```python
from build123d import *

# Parameters (mm, degrees)
F0_W      = 42
F0_H      = 13
F1_DEPTH  = 6
F2_W      = 17
F2_H      = 13
F5_DEPTH  = 27
F3_R      = 2.5
F6_DEPTH  = 6
F4_R      = 2.5
F7_DEPTH  = 6
F8_R      = 4
F9_DEPTH  = 15
F10_R     = 3.5
F11_DEPTH = 20
F12_W     = 1
F12_H     = 13
F13_DEPTH = 13


with BuildPart() as f1:
    # F0 (on Top) → F1 (new body)
    with BuildSketch(Plane.XY):
        Rectangle(F0_W, F0_H)
    extrude(amount=-F1_DEPTH)

    # F2 (on Top) → F5 (join)
    with BuildSketch(Plane.XY):
        Rectangle(F2_W, F2_H)
    extrude(amount=F5_DEPTH)

    # F3 (on Top) → F6 (cut)
    with BuildSketch(Plane.XY):
        with Locations((14.75, 0)):
            Circle(F3_R)
    extrude(amount=-F6_DEPTH, mode=Mode.SUBTRACT)

    # F4 (on Top) → F7 (cut)
    with BuildSketch(Plane.XY):
        with Locations((-14.75, 0)):
            Circle(F4_R)
    extrude(amount=-F7_DEPTH, mode=Mode.SUBTRACT)

    # F8 (on face) → F9 (cut)
    with BuildSketch(Plane.XZ.offset(6.5)):
        with Locations((0, 13.5)):
            Circle(F8_R)
    extrude(amount=-F9_DEPTH, mode=Mode.SUBTRACT)

    # F10 (on face) → F11 (cut)
    with BuildSketch(Plane.YZ.offset(8.5)):
        with Locations((0, 19)):
            Circle(F10_R)
    extrude(amount=-F11_DEPTH, mode=Mode.SUBTRACT)

    # F12 (on face) → F13 (cut)
    with BuildSketch(Plane.XY.offset(27)):
        Rectangle(F12_W, F12_H)
    extrude(amount=-F13_DEPTH, mode=Mode.SUBTRACT)


solid = f1.part
```
Geometry: final body of the model. Coordinates: model frame, mm. A direction names the side the tool comes from. Give positions to 0.01 mm unless a question says otherwise; leave off trailing zeros. Loops run counter-clockwise (first coordinate to the right, second up) from the corner with the lowest first, then second, coordinate; pieces in that order, holes last. Notation, with made-up numbers: (73, 27) -> (124, 27) arc R23 ccw to (124, 57) -> close; hole circle Ø6 at (3.5, -6.75). An arc over 180 degrees is marked (long way). Use one line per item in the form item = value.
Item 1: Section query D-D on z = 19. Output: boundary loops of the cut face in (x, y), and give its area (3 significant figures).
A:
outline = (-8.5, -6.5) -> (-0.5, -6.5) -> (-0.5, -3.5) -> (-8.5, -3.5) -> close; (-8.5, 3.5) -> (-0.5, 3.5) -> (-0.5, 6.5) -> (-8.5, 6.5) -> close; (0.5, -6.5) -> (8.5, -6.5) -> (8.5, -3.5) -> (0.5, -3.5) -> close; (0.5, 3.5) -> (8.5, 3.5) -> (8.5, 6.5) -> (0.5, 6.5) -> close
area = 96.0 mm^2
Item 2: Pin query (flat end, axial travel): P1, Ø2, axis at y = 2.5, z = 17.5, coming from the +X side; P2, Ø4, axis at x = 15.5, y = 0, coming from the +Z side; P3, Ø6.5, axis at y = 0.5, z = 16, coming from the -X side. Return the tip coordinate at first contact, or that it passes through.
A:
P1 = 8.5
P2 = 0
P3 = -8.5
Item 3: Line query: probe 1 along Y at (x, z) = (-14.75, -1.95); probe 2 along X at (y, z) = (1.75, 25.5); probe 3 along Z at (x, y) = (5, 0). Output: solid intervals per line, ascending.
A:
probe_1 = -6.5 to -2.5, 2.5 to 6.5
probe_2 = -8.5 to -0.5, 0.5 to 8.5
probe_3 = -6 to 15.5, 22.5 to 27
Item 4: Draft query along X for faces 1 (the face through (4.56, -0.46, 22.47)), 2 (the face through (8.5, 0, 13)), 3 (the face through (-0.5, 0, 23)), 4 (the face through (-17.248, 0.11, -2.958)). Return one class per face: pulls with the +X half, pulls with the -X half, needs draft (parallel to the pull), parting line crosses it, or undercut.
A:
face_1 = needs draft
face_2 = pulls with the +X half
face_3 = undercut
face_4 = undercut
Item 5: Access query for faces 5 (the face through (0.5, 0, 23)), 6 (the face through (-18, 0, 0)), 7 (the face through (12, 0, 0)), 8 (the face through (21, 0, -3)). Directions: +Z, -Z, +X, -X, +Y, -Y. A direction counts if a zero-diameter tool reaches every point of the face in a straight line with its end or side. Return the directions, or none.
A:
face_5 = +Z, +Y, -Y
face_6 = +Z, -X, +Y, -Y
face_7 = +Z, +X, +Y, -Y
face_8 = +Z, -Z, +X, +Y, -Y
Item 6: Section query B-B on x = 14.75. Output: boundary loops of the cut face in (y, z), and give its area (3 significant figures).
A:
outline = (-6.5, -6) -> (-2.5, -6) -> (-2.5, 0) -> (-6.5, 0) -> close; (2.5, -6) -> (6.5, -6) -> (6.5, 0) -> (2.5, 0) -> close
area = 48.0 mm^2
Item 7: Section query C-C on y = -1.5. Output: boundary loops of the cut face in (x, z).
A:
outline = (-21, -6) -> (-16.75, -6) -> (-16.75, 0) -> (-21, 0) -> close; (-12.75, -6) -> (12.75, -6) -> (12.75, 0) -> (8.5, 0) -> (8.5, 15.84) -> (3.25, 15.84) arc R4 cw (long way) to (-3.25, 15.84) -> (-8.5, 15.84) -> (-8.5, 0) -> (-12.75, 0) -> close; (-8.5, 22.16) -> (-0.5, 22.16) -> (-0.5, 27) -> (-8.5, 27) -> close; (0.5, 22.16) -> (8.5, 22.16) -> (8.5, 27) -> (0.5, 27) -> close; (16.75, -6) -> (21, -6) -> (21, 0) -> (16.75, 0) -> close
Item 8: Section query A-A on z = 13.5. Output: boundary loops of the cut face in (x, y), and give its area (3 significant figures).
A:
outline = (-8.5, -6.5) -> (-4, -6.5) -> (-4, 6.5) -> (-8.5, 6.5) -> close; (4, -6.5) -> (8.5, -6.5) -> (8.5, 6.5) -> (4, 6.5) -> close
area = 117 mm^2
